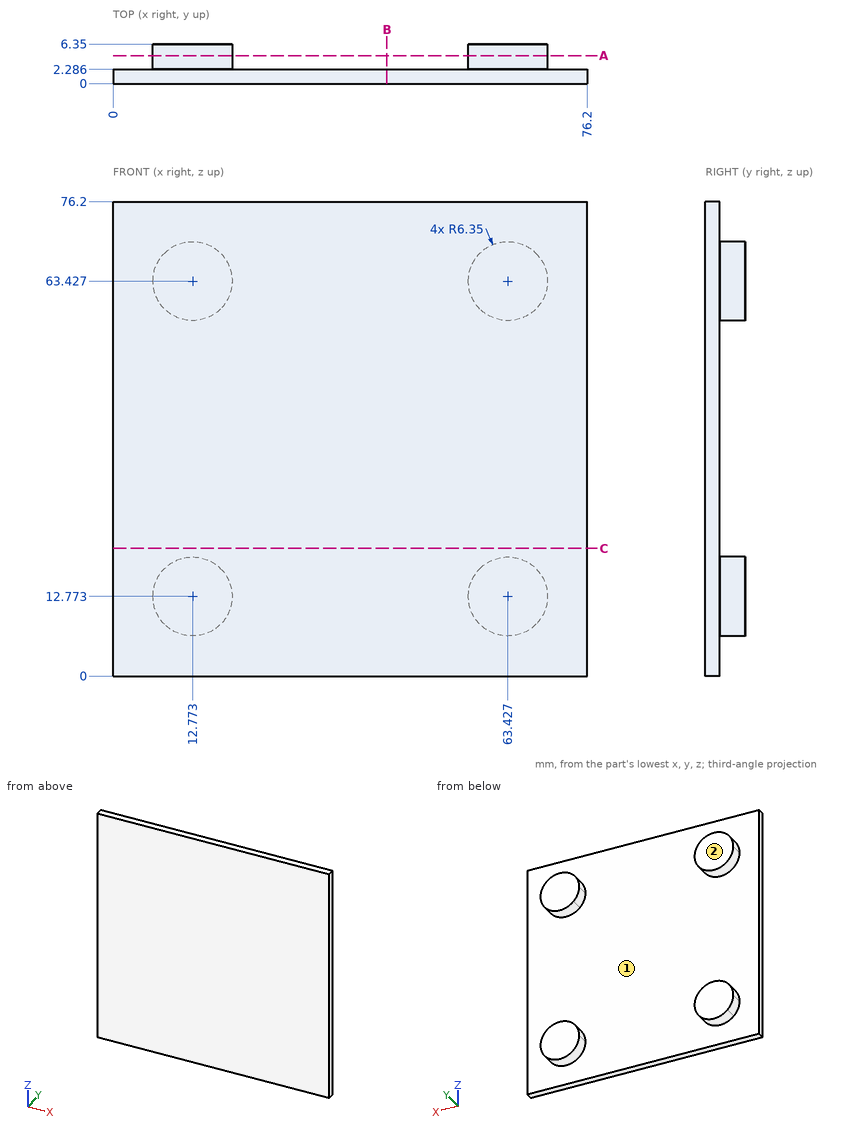
Geometry check sheet. Reference: drawing and pictorial views, mm from the part's lowest x, y, z. Round coordinates to 2 decimals unless told otherwise and drop trailing zeros. Loops run counter-clockwise (first coordinate to the right, second up) from the corner with the lowest first, then second, coordinate; pieces in that order, holes last.
1. Scan lines: probe 1 along Y at (x, z) = (29, 37.5); probe 2 along X at (y, z) = (2.5, 60.5); probe 3 along Z at (x, y) = (12, 2.75). Record each from-to range of solid material in increasing order.
2. Mould release check, pull along X, two halves, no side actions. Record for the marked faces 1 and 2: released by +X, released by -X, zero draft, split by the parting line, or undercut.
3. Sectioned sample at C-C on z = 20.5. Record the boundary of the cut face in (x, y).
4. Sectioned sample at A-A on y = 4.5. Record the boundary of the cut face in (x, z).
5. Gauge pin test, flat ends, axial feed: pin 1 Ø4 at (x, z) = (52, 14) entering from +Y; pin 2 Ø2 at (x, y) = (12.5, 5) entering from +Z. Record the tip position at first contact, or that the pin passes through.
6. Sectioned sample at B-B on x = 44. Record the boundary of the cut face in (y, z), and give its area (3 significant figures).
Recorded:
1. probe 1: y = 0 to 2.29
1. probe 2: x = 7.14 to 18.41, 57.79 to 69.06
1. probe 3: z = 6.47 to 19.08, 57.12 to 69.73
2. face 1: undercut
2. face 2: zero draft
3. outline: (0, 0) - (76.2, 0) - (76.2, 2.29) - (0, 2.29) - close
4. outline: circle Ø12.7 at (12.77, 12.77); circle Ø12.7 at (12.77, 63.43); circle Ø12.7 at (63.43, 12.77); circle Ø12.7 at (63.43, 63.43)
5. pin 1: stops at y = 2.29
5. pin 2: stops at z = 69.78
6. outline: (0, 0) - (2.29, 0) - (2.29, 76.2) - (0, 76.2) - close
6. area: 174 mm2
